For this review, take the finished solid that the model builds, in its own axes (mm). A direction names the side the tool comes from. Coordinates: 2 decimals unless noted, no trailing zeros. Order: outer loops, then holes, each group sorted by start corner. A loop starts at its lowest first (then second) coordinate and runs counter-clockwise, first axis right, second up. Notation, with made-up numbers: (58.5, 33) -> (89.5, 33) arc R9 cw to (89.5, 41) -> close; hole circle Ø10 at (-34.5, -24). An arc over 180 degrees is marked (long way). Answer as a JSON object with one key per item and string values. Group by question number.
1) Machinability: for faces 1 (the flat face through (301, 49.184, 39)), 2 (the cylindrical face through (317.392, 606.154, 23.747)), which of the approach directions +Z, -Z, +X, -X, +Y, -Y give a long, thin tool a straight path to every point of the face, cutting with its end or side? Answer none if there is none.
2) Add section B-B, the plane x = 304.8. Count the separate pieces of the cut face and the enclosed holes in it, then the cut area to 3 significant figures.
3) Wall thickness on L1, parallel to X at y = 409.5, z = 39; L2, parallel to Y at x = 371, z = 37; L3, parallel to X at y = 113.5, z = 5.5: over which ranges is each line inside the solid? List them lowest first.
4) Draft analysis for pull direction X (two halves, no side actions). For faces 3 (the cylindrical face through (317.392, 562.733, 23.747)), 4 (the flat face through (36.49, 305, 9)), 5 (the cylindrical face through (-11.61, 317.2, 22.65)), 6 (the flat face through (-16.763, 301, 42)), state which applies: +X half, -X half, draft (parallel to the pull), parting line (faces both ways), or undercut.
5) Add section A-A, the plane y = 452. Write out the cut boundary in (x, z), then the cut area to 3 significant figures.
from build123d import *

# Parameters (mm, degrees)
SKETCH1_W            = 643.125455594
SKETCH1_H            = 612.725254334
BOSS_EXTRUDE1_DEPTH  = 50.8
SKETCH3_W            = 536.564550572
SKETCH3_H            = 498.238511246
CUT_EXTRUDE2_DEPTH   = 50.8
SHELL5_START         = -6.602727797
SHELL5_OUTLINE_W     = 40.586297515
SHELL5_OUTLINE_H     = 30.48
SHELL5_OUTLINE_W_2   = 33.260445573
SHELL5_DEPTH         = 622.805455594
SHELL5_START_2       = 583.214532361
SHELL5_2_OUTLINE_W   = 518.558511246
SHELL5_2_OUTLINE_H   = 30.48
SHELL5_2_DEPTH       = 32.988195436
SHELL5_3_OUTLINE_W   = 518.558511246
SHELL5_3_OUTLINE_H   = 30.48
SHELL5_3_DEPTH       = 32.932709586
SKETCH7_W            = 66.675404896
SKETCH7_H            = 27.093969604
CUT_EXTRUDE3_DEPTH   = 50.8
LPATTERN1_COUNT      = 4
LPATTERN1_PITCH      = 151.6
LPATTERN1_COUNT_DIR2 = 2
LPATTERN1_PITCH_DIR2 = 553.72
SKETCH8_W            = 22.902108828
SKETCH8_H            = 56.707978581
CUT_EXTRUDE4_DEPTH   = 50.8
LPATTERN2_COUNT      = 4
LPATTERN2_PITCH      = 141.44
LPATTERN2_COUNT_DIR2 = 2
LPATTERN2_PITCH_DIR2 = 591.82
SKETCH11_R           = 12.7
CUT_EXTRUDE5_DEPTH   = 635
SKETCH12_R           = 12.7
CUT_EXTRUDE7_DEPTH   = 660.4


# Read off the part's stored shape, not the designer's step: Shell5
with BuildPart() as part:
    # Sketch1 → Boss-Extrude1 (new body)
    with BuildSketch(Plane.XY):
        with Locations((304.8, 304.8)):
            Rectangle(SKETCH1_W, SKETCH1_H)
    extrude(amount=BOSS_EXTRUDE1_DEPTH)

    # Sketch3 → Cut-Extrude2 (cut)
    with BuildSketch(Plane.XY.offset(50.8)):
        with Locations((304.772257075, 308.462925971)):
            Rectangle(SKETCH3_W, SKETCH3_H)
    extrude(amount=-CUT_EXTRUDE2_DEPTH, mode=Mode.SUBTRACT)

    # Shell5 outline → Shell5 (cut)
    with BuildSketch(Plane.YZ.offset(SHELL5_START)):
        with Locations((28.890521591, 25.4)):
            Rectangle(SHELL5_OUTLINE_W, SHELL5_OUTLINE_H)
        with Locations((584.372404381, 25.4)):
            Rectangle(SHELL5_OUTLINE_W_2, SHELL5_OUTLINE_H)
    extrude(amount=SHELL5_DEPTH, mode=Mode.SUBTRACT)

    # Shell5 2 outline → Shell5 2 (cut)
    with BuildSketch(Plane.YZ.offset(SHELL5_START_2)):
        with Locations((308.462925971, 25.4)):
            Rectangle(SHELL5_2_OUTLINE_W, SHELL5_2_OUTLINE_H)
    extrude(amount=SHELL5_2_DEPTH, mode=Mode.SUBTRACT)

    # Shell5 3 outline → Shell5 3 (cut)
    with BuildSketch(Plane.YZ.offset(SHELL5_START)):
        with Locations((308.462925971, 25.4)):
            Rectangle(SHELL5_3_OUTLINE_W, SHELL5_3_OUTLINE_H)
    extrude(amount=SHELL5_3_DEPTH, mode=Mode.SUBTRACT)

    # Sketch7 → Cut-Extrude3 (cut)
    with BuildSketch(Plane.XY.offset(50.8)):
        with Locations((76.34692027, 584.240607078)):
            Rectangle(SKETCH7_W, SKETCH7_H)
    cut_extrude3 = extrude(amount=-CUT_EXTRUDE3_DEPTH, mode=Mode.SUBTRACT)

    # LPattern1: Cut-Extrude3 4 × 2
    with Locations(*[(i * LPATTERN1_PITCH, -j * LPATTERN1_PITCH_DIR2, 0) for i in range(LPATTERN1_COUNT) for j in range(LPATTERN1_COUNT_DIR2) if (i, j) != (0, 0)]):
        add(cut_extrude3, mode=Mode.SUBTRACT)

    # Sketch8 → Cut-Extrude4 (cut)
    with BuildSketch(Plane.XY.offset(50.8)):
        with Locations((9.129138523, 525.334860242)):
            Rectangle(SKETCH8_W, SKETCH8_H)
    cut_extrude4 = extrude(amount=-CUT_EXTRUDE4_DEPTH, mode=Mode.SUBTRACT)

    # LPattern2: Cut-Extrude4 4 × 2
    with Locations(*[(j * LPATTERN2_PITCH_DIR2, -i * LPATTERN2_PITCH, 0) for i in range(LPATTERN2_COUNT) for j in range(LPATTERN2_COUNT_DIR2) if (i, j) != (0, 0)]):
        add(cut_extrude4, mode=Mode.SUBTRACT)

    # Sketch11 → Cut-Extrude5 (cut)
    with BuildSketch(Plane(origin=(0, 611.162627167, 0), x_dir=(1, 0, 0), z_dir=(0, 1, 0))):
        with Locations(Location((304.8, -25.4, 0), (0, 0, 270))):
            Circle(SKETCH11_R)
    extrude(amount=-CUT_EXTRUDE5_DEPTH, mode=Mode.SUBTRACT)

    # Sketch12 → Cut-Extrude7 (cut)
    with BuildSketch(Plane(origin=(626.362727797, 0, 0), x_dir=(0, 0, -1), z_dir=(1, 0, 0))):
        with Locations(Location((-25.4, 304.8, 0), (0, 0, 180))):
            Circle(SKETCH12_R)
    extrude(amount=-CUT_EXTRUDE7_DEPTH, mode=Mode.SUBTRACT)


solid = part.part
Output values:
{
 "1": {"face 1": "none", "face 2": "+Y, -Y"},
 "2": {"separate pieces": "4", "enclosed holes": "0", "area": "2,530 mm²"},
 "3": {"L1": "x = -16.76 to -6.6, 26.33 to 36.49, 573.05 to 583.21, 616.2 to 626.36", "L2": "y = -1.56 to 8.6, 49.18 to 59.34, 557.58 to 567.74, 601 to 611.16", "L3": "x = -16.76 to -2.32, 20.58 to 36.49, 573.05 to 589.5, 612.4 to 626.36"},
 "4": {"face 3": "undercut", "face 4": "undercut", "face 5": "draft", "face 6": "-X half"},
 "5": {"outline": "(-16.76, 0) -> (36.49, 0) -> (36.49, 50.8) -> (-16.76, 50.8) -> close; (573.05, 0) -> (626.36, 0) -> (626.36, 50.8) -> (573.05, 50.8) -> close; hole (-6.6, 10.16) -> (26.33, 10.16) -> (26.33, 40.64) -> (-6.6, 40.64) -> close; hole (583.21, 10.16) -> (616.2, 10.16) -> (616.2, 40.64) -> (583.21, 40.64) -> close", "area": "3,400 mm²"}
}
